Source: CAD feature listing. Evaluate the final solid. Frame: model axes, mm. Give positions to 0.01 mm unless a question says otherwise; leave off trailing zeros. Order: outer loops, then holes, each group sorted by start corner. A loop starts at its lowest first (then second) coordinate and runs counter-clockwise, first axis right, second up.
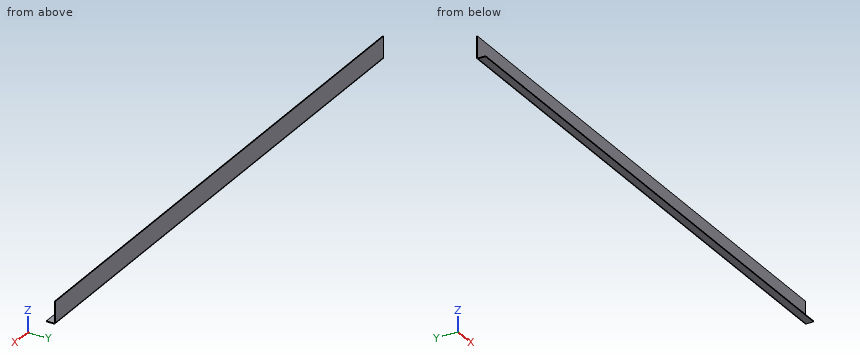
Autodesk Inventor part; units mm, degrees
ref_plane "YZ Plane" through (0, 0, 0) normal (1, 0, 0) x (0, 1, 0)
ref_plane "XZ Plane" through (0, 0, 0) normal (0, 1, 0) x (-1, 0, 0)
ref_plane "XY Plane" through (0, 0, 0) normal (0, 0, 1) x (1, 0, 0)
sketch "Sketch3" plane through (0, 0, 0) normal (0, 1, 0) x (-1, 0, 0)
  line L0 (0, 0) -> (-1200, 0)
  line L1 (-1200, 0) -> (-1200, -50)
  line L2 (-1200, -50) -> (0, -50)
  line L3 (0, -50) -> (0, 0)
  dimension "d25" = 50
  dimension "d28" = 1200
extrude "Plate3" add sketch "Sketch3" along normal blind 2
sketch "Sketch4" plane through (1200, 2, -48) normal (0, 0, -1) x (-1, 0, 0)
  line L0 (1200, 0) -> (0, 0)
  line L1 (0, 0) -> (0, -20)
  line L2 (0, -20) -> (1200, -20)
  line L3 (1200, -20) -> (1200, 0)
edge flange "Flange2" height 20 angle 90 thickness 2 bend radius 2 thickness toward (0, 0, -1) relief tear relief width 2 relief depth 1 edges at (600, 0, -50) wall of the first edge with corners at (0, 2, -48) (1200, 2, -48) (1200, -18, -48) (0, -18, -48)
bend "Bend3"
corner "Corner3"
equation "\"d30\" = Thickness"
equation "\"d31\" = BendReliefWidth"
equation "\"d32\" = BendReliefDepth"
equation "\"d33\" = MinimumRemnant"
equation "\"d34\" = TransitionRadius"
equation "\"d37\" = BendRadius"
equation "\"d38\" = CornerReliefSize"
equation "\"d39\" = GapSize"
equation "\"d40\" = JacobiRadiusSize"
equation "\"BendRadius\" = Thickness"
equation "\"BendReliefWidth\" = Thickness"
equation "\"BendReliefDepth\" = 0.5 * Thickness"
equation "\"CornerReliefSize\" = 4 * Thickness"
equation "\"MinimumRemnant\" = 2 * Thickness"
equation "\"TransitionRadius\" = BendRadius"
equation "\"JacobiRadiusSize\" = BendRadius"
equation "\"GapSize\" = Thickness"
properties part number "GBK-RK-0042 rib 2"
1) Material intervals for L1, parallel to Y at x = 1042, z = -23.5; L2, parallel to Z at x = 229, y = -12.5; L3, parallel to Z at x = 450, y = -0.5, sorted ascending.
Report:
L1: y = 0 to 2
L2: z = -50 to -48
L3: z = -49.71 to -47.32
2) Section query C-C, the plane z = -19.5. Return the cut outline in (x, y), and give its area (3 significant figures).
Report:
outline: (0, 0) - (1200, 0) - (1200, 2) - (0, 2) - close
area: 2,400 mm2
3) Section query A-A, the plane x = 539.5. Return the cut outline in (y, z).
Report:
outline: (-18, -50) - (-2, -50) arc R4 ccw to (2, -46) - (2, 0) - (0, 0) - (0, -46) arc R2 cw to (-2, -48) - (-18, -48) - close
4) Pin query (flat end, axial travel): pin 1 (8 mm diameter, centred on x = 689, y = -9, fed in from +Z); pin 2 (23 mm diameter, centred on x = 759.5, z = -27.5, fed in from -Y). Return the tip coordinate at first contact, or that it passes through.
Report:
pin 1: stops at z = -48
pin 2: stops at y = 0
5) Section query B-B, the plane y = -5.25. Return the cut outline in (x, z), and give its area (3 significant figures).
Report:
outline: (0, -50) - (1200, -50) - (1200, -48) - (0, -48) - close
area: 2,400 mm2
